Work out the finished part from the listing and answer in its coordinate system (mm). Round coordinates to 2 decimals unless told otherwise and drop trailing zeros. Order: outer loops, then holes, each group sorted by start corner. A loop starts at its lowest first (then second) coordinate and runs counter-clockwise, first axis right, second up. Notation, with made-up numbers: (89.25, -13) - (128.25, -13) arc R17 cw to (128.25, -5) - close; hole circle Ø4 at (-29.5, 56.5). An arc over 180 degrees is marked (long way). One line per question, with ' | ' between items. Start each with the question number.
Autodesk Inventor part; units mm, degrees
ref_plane "YZ Plane" through (0, 0, 0) normal (1, 0, 0) x (0, 1, 0)
ref_plane "XZ Plane" through (0, 0, 0) normal (0, 1, 0) x (-1, 0, 0)
ref_plane "XY Plane" through (0, 0, 0) normal (0, 0, 1) x (1, 0, 0)
sketch "Sketch1" plane through (0, 0, 0) normal (0, 0, 1) x (1, 0, 0)
  circle A0 centre (-11.2222, 3.5185) radius 8
  point P0 (0, 0)
  dimension "d0" = 16
extrude "Extrusion1" add sketch "Sketch1" along normal blind 140
fillet "Fillet1" radius 3 2 edges at (-19.2222, 3.5185, 140) (-19.2222, 3.5185, 0)
sketch "Sketch2" plane through (0, 0, 0) normal (1, 0, 0) x (0, 1, 0)
  line L0 (-1.4815, 140) -> (8.5185, 140)
  line L1 (3.5185, 140) -> (3.5185, 40)
  circle A0 centre (3.5185, 133) radius 2.5
  circle A1 centre (3.5185, 7) radius 2.5
  line L2 (8.5185, 0) -> (-1.4815, 0)
  point P0 (0, 0)
  dimension "d4" = 5
  dimension "d5" = 5
  dimension "d6" = 7
  dimension "d10" = 7
extrude "Extrusion2" cut sketch "Sketch2" against normal blind 100
properties part number "Eixo_16mm" material "SAE 1010/1020"
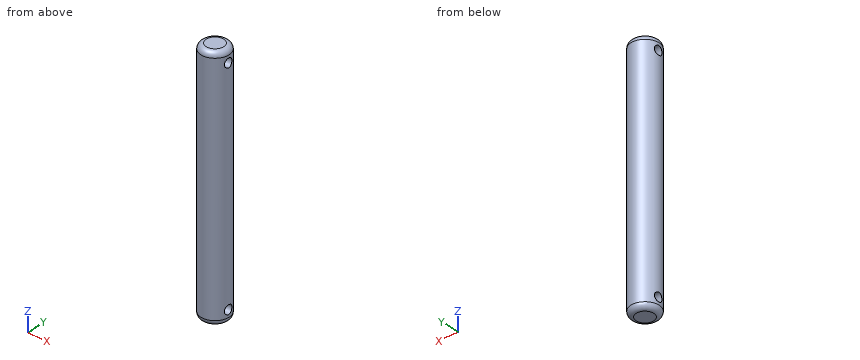
1) Section A-A on z = 7 is taken. Give the vertices of the cut face in (x, y), and give its area (3 significant figures).
2) Straight lines are drawn through the part: line 1 (Z direction, x = -11.75, y = 4.25); line 2 (Z direction, x = -17.25, y = 4.75); line 3 (Y direction, x = -8.5, z = 7). For each, find the intervals that lie inside material, in ascending order.
3) Section C-C on z = 117 is taken. Give the vertices of the cut face in (x, y).
4) Flat-ended cylindrical pins translate along their axes: pin 1 (4 mm diameter, centred on y = 3.52, z = 133, fed in from +X); pin 2 (1 mm diameter, centred on x = -9, z = 124, fed in from +Y); pin 3 (8 mm diameter, centred on y = 9, z = 65, fed in from -X); pin 4 (1.5 mm diameter, centred on x = -16.5, z = 30, fed in from +Y). Find the tip coordinate at first contact, or state that the pin passes through.
5) Section B-B on x = -13.5 is taken. Give the number of separate pieces and of enclosed holes in the cut face, and give its area (3 significant figures).
Recorded:
1) outline: (-18.82, 1.02) arc R8 ccw to (-3.62, 1.02) - close; (-18.82, 6.02) - (-3.62, 6.02) arc R8 ccw to start | area: 122 mm²
2) line 1: z = 0 to 4.61, 9.39 to 130.61, 135.39 to 140 | line 2: z = 0.23 to 4.82, 9.18 to 130.82, 135.18 to 139.77 | line 3: y = -4 to 1.02, 6.02 to 11.04
3) outline: circle Ø16 at (-11.22, 3.52)
4) pin 1: passes through | pin 2: stops at y = 11.33 | pin 3: stops at x = -19.08 | pin 4: stops at y = 10.11
5) separate pieces: 1 | enclosed holes: 2 | area: 2,100 mm²
